Geometry: final body of the model. Coordinates: model frame, mm. Face numbers are marked on the shaded views. A direction names the side the tool comes from. Coordinates: 2 decimals unless noted, no trailing zeros. Write each loop counter-clockwise with the first axis right and the second up, starting at its lowest first coordinate (ties: lowest second). Pieces come first, ordered by that corner, then holes. Notation, with made-up numbers: (28, 46) -> (47, 46) arc R28 ccw to (47, 82) -> close; hole circle Ø3 at (32.5, 20). An arc over 180 degrees is marked (long way). One line per item, written item: value.
Autodesk Inventor part; units mm, degrees
ref_plane "YZ Plane" through (0, 0, 0) normal (1, 0, 0) x (0, 1, 0)
ref_plane "XZ Plane" through (0, 0, 0) normal (0, 1, 0) x (-1, 0, 0)
ref_plane "XY Plane" through (0, 0, 0) normal (0, 0, 1) x (1, 0, 0)
sketch "Sketch1" plane through (0, 0, 0) normal (1, 0, 0) x (0, 1, 0)
  arc A0 (-4.3875, 5.1282) -> (-5.1282, 4.3875) centre (0, 0) ccw
  arc A1 (-5.1895, 7.3532) -> (-4.3875, 5.1282) centre (-1.9912, 7.249) ccw
  arc A2 (-3.0589, 6.016) -> (-4.8075, 7.6084) centre (-5.9352, 4.6137) ccw
  arc A3 (-4.8075, 7.6084) -> (-5.1895, 7.3532) centre (0, 0) ccw
  arc A4 (-2.091, 6.4169) -> (-3.0589, 6.016) centre (0, 0) ccw
  arc A5 (-1.9805, 8.7794) -> (-2.091, 6.4169) centre (0.9345, 7.4592) ccw
  arc A6 (-1.5299, 8.869) -> (-1.9805, 8.7794) centre (0, 0) ccw
  arc A7 (-0.5238, 6.7286) -> (-1.5299, 8.869) centre (-3.7179, 6.5338) ccw
  arc A8 (0.5238, 6.7286) -> (-0.5238, 6.7286) centre (0, 0) ccw
  arc A9 (1.5299, 8.869) -> (0.5238, 6.7286) centre (3.7179, 6.5338) ccw
  arc A10 (1.9805, 8.7794) -> (1.5299, 8.869) centre (0, 0) ccw
  arc A11 (2.091, 6.4169) -> (1.9805, 8.7794) centre (-0.9345, 7.4592) ccw
  arc A12 (3.0589, 6.016) -> (2.091, 6.4169) centre (0, 0) ccw
  arc A13 (4.8075, 7.6084) -> (3.0589, 6.016) centre (5.9352, 4.6137) ccw
  arc A14 (5.1895, 7.3532) -> (4.8075, 7.6084) centre (0, 0) ccw
  arc A15 (4.3875, 5.1282) -> (5.1895, 7.3532) centre (1.9912, 7.249) ccw
  arc A16 (5.1282, 4.3875) -> (4.3875, 5.1282) centre (0, 0) ccw
  arc A17 (7.3532, 5.1895) -> (5.1282, 4.3875) centre (7.249, 1.9912) ccw
  arc A18 (7.6084, 4.8075) -> (7.3532, 5.1895) centre (0, 0) ccw
  arc A19 (6.016, 3.0589) -> (7.6084, 4.8075) centre (4.6137, 5.9352) ccw
  arc A20 (6.4169, 2.091) -> (6.016, 3.0589) centre (0, 0) ccw
  arc A21 (8.7794, 1.9805) -> (6.4169, 2.091) centre (7.4592, -0.9345) ccw
  arc A22 (8.869, 1.5299) -> (8.7794, 1.9805) centre (0, 0) ccw
  arc A23 (6.7286, 0.5238) -> (8.869, 1.5299) centre (6.5338, 3.7179) ccw
  arc A24 (6.7286, -0.5238) -> (6.7286, 0.5238) centre (0, 0) ccw
  arc A25 (8.869, -1.5299) -> (6.7286, -0.5238) centre (6.5338, -3.7179) ccw
  arc A26 (8.7794, -1.9805) -> (8.869, -1.5299) centre (0, 0) ccw
  arc A27 (6.4169, -2.091) -> (8.7794, -1.9805) centre (7.4592, 0.9345) ccw
  arc A28 (6.016, -3.0589) -> (6.4169, -2.091) centre (0, 0) ccw
  arc A29 (7.6084, -4.8075) -> (6.016, -3.0589) centre (4.6137, -5.9352) ccw
  arc A30 (7.3532, -5.1895) -> (7.6084, -4.8075) centre (0, 0) ccw
  arc A31 (5.1282, -4.3875) -> (7.3532, -5.1895) centre (7.249, -1.9912) ccw
  arc A32 (4.3875, -5.1282) -> (5.1282, -4.3875) centre (0, 0) ccw
  arc A33 (5.1895, -7.3532) -> (4.3875, -5.1282) centre (1.9912, -7.249) ccw
  arc A34 (4.8075, -7.6084) -> (5.1895, -7.3532) centre (0, 0) ccw
  arc A35 (3.0589, -6.016) -> (4.8075, -7.6084) centre (5.9352, -4.6137) ccw
  arc A36 (-8.869, 1.5299) -> (-6.7286, 0.5238) centre (-6.5338, 3.7179) ccw
  arc A37 (-6.7286, 0.5238) -> (-6.7286, -0.5238) centre (0, 0) ccw
  arc A38 (-6.7286, -0.5238) -> (-8.869, -1.5299) centre (-6.5338, -3.7179) ccw
  arc A39 (-8.869, -1.5299) -> (-8.7794, -1.9805) centre (0, 0) ccw
  arc A40 (-8.7794, -1.9805) -> (-6.4169, -2.091) centre (-7.4592, 0.9345) ccw
  arc A41 (-6.4169, -2.091) -> (-6.016, -3.0589) centre (0, 0) ccw
  arc A42 (-6.016, -3.0589) -> (-7.6084, -4.8075) centre (-4.6137, -5.9352) ccw
  arc A43 (-7.6084, -4.8075) -> (-7.3532, -5.1895) centre (0, 0) ccw
  arc A44 (-7.3532, -5.1895) -> (-5.1282, -4.3875) centre (-7.249, -1.9912) ccw
  arc A45 (-5.1282, -4.3875) -> (-4.3875, -5.1282) centre (0, 0) ccw
  arc A46 (-4.3875, -5.1282) -> (-5.1895, -7.3532) centre (-1.9912, -7.249) ccw
  arc A47 (-5.1895, -7.3532) -> (-4.8075, -7.6084) centre (0, 0) ccw
  arc A48 (-4.8075, -7.6084) -> (-3.0589, -6.016) centre (-5.9352, -4.6137) ccw
  arc A49 (-3.0589, -6.016) -> (-2.091, -6.4169) centre (0, 0) ccw
  arc A50 (-2.091, -6.4169) -> (-1.9805, -8.7794) centre (0.9345, -7.4592) ccw
  arc A51 (-1.9805, -8.7794) -> (-1.5299, -8.869) centre (0, 0) ccw
  arc A52 (-1.5299, -8.869) -> (-0.5238, -6.7286) centre (-3.7179, -6.5338) ccw
  arc A53 (-0.5238, -6.7286) -> (0.5238, -6.7286) centre (0, 0) ccw
  arc A54 (0.5238, -6.7286) -> (1.5299, -8.869) centre (3.7179, -6.5338) ccw
  arc A55 (1.5299, -8.869) -> (1.9805, -8.7794) centre (0, 0) ccw
  arc A56 (1.9805, -8.7794) -> (2.091, -6.4169) centre (-0.9345, -7.4592) ccw
  arc A57 (2.091, -6.4169) -> (3.0589, -6.016) centre (0, 0) ccw
  arc A58 (3.0589, -6.016) -> (4.8075, -7.6084) centre (5.9352, -4.6137) ccw
  arc A59 (4.8075, -7.6084) -> (5.1895, -7.3532) centre (0, 0) ccw
  arc A60 (5.1895, -7.3532) -> (4.3875, -5.1282) centre (1.9912, -7.249) ccw
  arc A61 (4.3875, -5.1282) -> (5.1282, -4.3875) centre (0, 0) ccw
  arc A62 (5.1282, -4.3875) -> (7.3532, -5.1895) centre (7.249, -1.9912) ccw
  arc A63 (7.3532, -5.1895) -> (7.6084, -4.8075) centre (0, 0) ccw
  arc A64 (7.6084, -4.8075) -> (6.016, -3.0589) centre (4.6137, -5.9352) ccw
  arc A65 (6.016, -3.0589) -> (6.4169, -2.091) centre (0, 0) ccw
  arc A66 (6.4169, -2.091) -> (8.7794, -1.9805) centre (7.4592, 0.9345) ccw
  arc A67 (8.7794, -1.9805) -> (8.869, -1.5299) centre (0, 0) ccw
  arc A68 (8.869, -1.5299) -> (6.7286, -0.5238) centre (6.5338, -3.7179) ccw
  arc A69 (6.7286, -0.5238) -> (6.7286, 0.5238) centre (0, 0) ccw
  arc A70 (6.7286, 0.5238) -> (8.869, 1.5299) centre (6.5338, 3.7179) ccw
  arc A71 (8.869, 1.5299) -> (8.7794, 1.9805) centre (0, 0) ccw
  arc A72 (8.7794, 1.9805) -> (6.4169, 2.091) centre (7.4592, -0.9345) ccw
  arc A73 (6.4169, 2.091) -> (6.016, 3.0589) centre (0, 0) ccw
  arc A74 (6.016, 3.0589) -> (7.6084, 4.8075) centre (4.6137, 5.9352) ccw
  arc A75 (7.6084, 4.8075) -> (7.3532, 5.1895) centre (0, 0) ccw
  arc A76 (7.3532, 5.1895) -> (5.1282, 4.3875) centre (7.249, 1.9912) ccw
  arc A77 (5.1282, 4.3875) -> (4.3875, 5.1282) centre (0, 0) ccw
  arc A78 (4.3875, 5.1282) -> (5.1895, 7.3532) centre (1.9912, 7.249) ccw
  arc A79 (5.1895, 7.3532) -> (4.8075, 7.6084) centre (0, 0) ccw
  arc A80 (4.8075, 7.6084) -> (3.0589, 6.016) centre (5.9352, 4.6137) ccw
  arc A81 (3.0589, 6.016) -> (2.091, 6.4169) centre (0, 0) ccw
  arc A82 (2.091, 6.4169) -> (1.9805, 8.7794) centre (-0.9345, 7.4592) ccw
  arc A83 (1.9805, 8.7794) -> (1.5299, 8.869) centre (0, 0) ccw
  arc A84 (1.5299, 8.869) -> (0.5238, 6.7286) centre (3.7179, 6.5338) ccw
  arc A85 (0.5238, 6.7286) -> (-0.5238, 6.7286) centre (0, 0) ccw
  arc A86 (-0.5238, 6.7286) -> (-1.5299, 8.869) centre (-3.7179, 6.5338) ccw
  arc A87 (-1.5299, 8.869) -> (-1.9805, 8.7794) centre (0, 0) ccw
  arc A88 (-1.9805, 8.7794) -> (-2.091, 6.4169) centre (0.9345, 7.4592) ccw
  arc A89 (-2.091, 6.4169) -> (-3.0589, 6.016) centre (0, 0) ccw
  arc A90 (-3.0589, 6.016) -> (-4.8075, 7.6084) centre (-5.9352, 4.6137) ccw
  arc A91 (-4.8075, 7.6084) -> (-5.1895, 7.3532) centre (0, 0) ccw
  arc A92 (-5.1895, 7.3532) -> (-4.3875, 5.1282) centre (-1.9912, 7.249) ccw
  arc A93 (-4.3875, 5.1282) -> (-5.1282, 4.3875) centre (0, 0) ccw
  arc A94 (-5.1282, 4.3875) -> (-7.3532, 5.1895) centre (-7.249, 1.9912) ccw
  arc A95 (-7.3532, 5.1895) -> (-7.6084, 4.8075) centre (0, 0) ccw
  arc A96 (-7.6084, 4.8075) -> (-6.016, 3.0589) centre (-4.6137, 5.9352) ccw
  arc A97 (-6.016, 3.0589) -> (-6.4169, 2.091) centre (0, 0) ccw
  arc A98 (-6.4169, 2.091) -> (-8.7794, 1.9805) centre (-7.4592, -0.9345) ccw
  arc A99 (-8.7794, 1.9805) -> (-8.869, 1.5299) centre (0, 0) ccw
  circle A100 centre (0, 0) radius 2.5
  line L0 (0, 0) -> (2.25, 0)
  line L1 (-1.5245, 0) -> (0, 0)
  line L2 (0, 0) -> (0, -2.5981)
  point P0 (3.0589, -6.016)
  point P1 (-5.1282, 4.3875)
  dimension "d17" = 5
extrude "Extrusion1" add sketch "Sketch1" along normal blind 4.5
sketch "Sketch4" plane through (4.5, 0, 0) normal (1, 0, 0) x (0, 0, -1)
  circle A0 centre (0, 0) radius 1.5
  arc A1 (6.016, 3.0589) -> (7.6084, 4.8075) centre (4.6137, 5.9352) ccw
  arc A2 (7.6084, 4.8075) -> (7.3532, 5.1895) centre (0, 0) ccw
  arc A3 (7.3532, 5.1895) -> (5.1282, 4.3875) centre (7.249, 1.9912) ccw
  arc A4 (5.1282, 4.3875) -> (4.3875, 5.1282) centre (0, 0) ccw
  arc A5 (4.3875, 5.1282) -> (5.1895, 7.3532) centre (1.9912, 7.249) ccw
  arc A6 (5.1895, 7.3532) -> (4.8075, 7.6084) centre (0, 0) ccw
  arc A7 (4.8075, 7.6084) -> (3.0589, 6.016) centre (5.9352, 4.6137) ccw
  arc A8 (3.0589, 6.016) -> (2.091, 6.4169) centre (0, 0) ccw
  arc A9 (2.091, 6.4169) -> (1.9805, 8.7794) centre (-0.9345, 7.4592) ccw
  arc A10 (1.9805, 8.7794) -> (1.5299, 8.869) centre (0, 0) ccw
  arc A11 (1.5299, 8.869) -> (0.5238, 6.7286) centre (3.7179, 6.5338) ccw
  arc A12 (0.5238, 6.7286) -> (-0.5238, 6.7286) centre (0, 0) ccw
  arc A13 (-0.5238, 6.7286) -> (-1.5299, 8.869) centre (-3.7179, 6.5338) ccw
  arc A14 (-1.5299, 8.869) -> (-1.9805, 8.7794) centre (0, 0) ccw
  arc A15 (-1.9805, 8.7794) -> (-2.091, 6.4169) centre (0.9345, 7.4592) ccw
  arc A16 (-2.091, 6.4169) -> (-3.0589, 6.016) centre (0, 0) ccw
  arc A17 (-3.0589, 6.016) -> (-4.8075, 7.6084) centre (-5.9352, 4.6137) ccw
  arc A18 (-4.8075, 7.6084) -> (-5.1895, 7.3532) centre (0, 0) ccw
  arc A19 (-5.1895, 7.3532) -> (-4.3875, 5.1282) centre (-1.9912, 7.249) ccw
  arc A20 (-4.3875, 5.1282) -> (-5.1282, 4.3875) centre (0, 0) ccw
  arc A21 (-5.1282, 4.3875) -> (-7.3532, 5.1895) centre (-7.249, 1.9912) ccw
  arc A22 (-7.3532, 5.1895) -> (-7.6084, 4.8075) centre (0, 0) ccw
  arc A23 (-7.6084, 4.8075) -> (-6.016, 3.0589) centre (-4.6137, 5.9352) ccw
  arc A24 (-6.016, 3.0589) -> (-6.4169, 2.091) centre (0, 0) ccw
  arc A25 (-6.4169, 2.091) -> (-8.7794, 1.9805) centre (-7.4592, -0.9345) ccw
  arc A26 (-8.7794, 1.9805) -> (-8.869, 1.5299) centre (0, 0) ccw
  arc A27 (-8.869, 1.5299) -> (-6.7286, 0.5238) centre (-6.5338, 3.7179) ccw
  arc A28 (-6.7286, 0.5238) -> (-6.7286, -0.5238) centre (0, 0) ccw
  arc A29 (-6.7286, -0.5238) -> (-8.869, -1.5299) centre (-6.5338, -3.7179) ccw
  arc A30 (-8.869, -1.5299) -> (-8.7794, -1.9805) centre (0, 0) ccw
  arc A31 (-8.7794, -1.9805) -> (-6.4169, -2.091) centre (-7.4592, 0.9345) ccw
  arc A32 (-6.4169, -2.091) -> (-6.016, -3.0589) centre (0, 0) ccw
  arc A33 (-6.016, -3.0589) -> (-7.6084, -4.8075) centre (-4.6137, -5.9352) ccw
  arc A34 (-7.6084, -4.8075) -> (-7.3532, -5.1895) centre (0, 0) ccw
  arc A35 (-7.3532, -5.1895) -> (-5.1282, -4.3875) centre (-7.249, -1.9912) ccw
  arc A36 (-5.1282, -4.3875) -> (-4.3875, -5.1282) centre (0, 0) ccw
  arc A37 (-4.3875, -5.1282) -> (-5.1895, -7.3532) centre (-1.9912, -7.249) ccw
  arc A38 (-5.1895, -7.3532) -> (-4.8075, -7.6084) centre (0, 0) ccw
  arc A39 (-4.8075, -7.6084) -> (-3.0589, -6.016) centre (-5.9352, -4.6137) ccw
  arc A40 (-3.0589, -6.016) -> (-2.091, -6.4169) centre (0, 0) ccw
  arc A41 (-2.091, -6.4169) -> (-1.9805, -8.7794) centre (0.9345, -7.4592) ccw
  arc A42 (-1.9805, -8.7794) -> (-1.5299, -8.869) centre (0, 0) ccw
  arc A43 (-1.5299, -8.869) -> (-0.5238, -6.7286) centre (-3.7179, -6.5338) ccw
  arc A44 (-0.5238, -6.7286) -> (0.5238, -6.7286) centre (0, 0) ccw
  arc A45 (0.5238, -6.7286) -> (1.5299, -8.869) centre (3.7179, -6.5338) ccw
  arc A46 (1.5299, -8.869) -> (1.9805, -8.7794) centre (0, 0) ccw
  arc A47 (1.9805, -8.7794) -> (2.091, -6.4169) centre (-0.9345, -7.4592) ccw
  arc A48 (2.091, -6.4169) -> (3.0589, -6.016) centre (0, 0) ccw
  arc A49 (3.0589, -6.016) -> (4.8075, -7.6084) centre (5.9352, -4.6137) ccw
  arc A50 (4.8075, -7.6084) -> (5.1895, -7.3532) centre (0, 0) ccw
  arc A51 (5.1895, -7.3532) -> (4.3875, -5.1282) centre (1.9912, -7.249) ccw
  arc A52 (4.3875, -5.1282) -> (5.1282, -4.3875) centre (0, 0) ccw
  arc A53 (5.1282, -4.3875) -> (7.3532, -5.1895) centre (7.249, -1.9912) ccw
  arc A54 (7.3532, -5.1895) -> (7.6084, -4.8075) centre (0, 0) ccw
  arc A55 (7.6084, -4.8075) -> (6.016, -3.0589) centre (4.6137, -5.9352) ccw
  arc A56 (6.016, -3.0589) -> (6.4169, -2.091) centre (0, 0) ccw
  arc A57 (6.4169, -2.091) -> (8.7794, -1.9805) centre (7.4592, 0.9345) ccw
  arc A58 (8.7794, -1.9805) -> (8.869, -1.5299) centre (0, 0) ccw
  arc A59 (8.869, -1.5299) -> (6.7286, -0.5238) centre (6.5338, -3.7179) ccw
  arc A60 (6.7286, -0.5238) -> (6.7286, 0.5238) centre (0, 0) ccw
  arc A61 (6.7286, 0.5238) -> (8.869, 1.5299) centre (6.5338, 3.7179) ccw
  arc A62 (8.869, 1.5299) -> (8.7794, 1.9805) centre (0, 0) ccw
  arc A63 (8.7794, 1.9805) -> (6.4169, 2.091) centre (7.4592, -0.9345) ccw
  arc A64 (6.4169, 2.091) -> (6.016, 3.0589) centre (0, 0) ccw
  circle A65 centre (0, 0) radius 2.5
  circle A66 centre (0, 0) radius 3
  dimension "d18" = 3
  dimension "d19" = 6
extrude "Extrusion3" add sketch "Sketch4" along normal blind 2 contours A65 | A66
fillet "Fillet1" radius 1 1 edges at (4.5, 0, 3)
equation "\"d17\" = d_agu"
equation "\"d_agu\" = 5"
properties part number "engrane_v3"
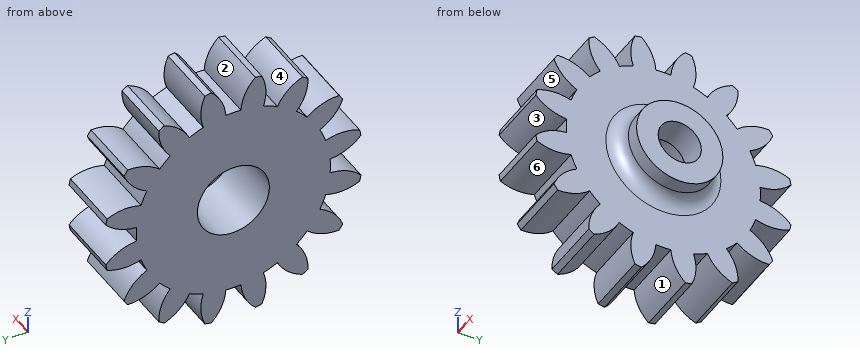
(1) Reachability of the marked faces 4, 5 and 6 from +Z, -Z, +X, -X, +Y, -Y: full face, straight path, thin tool, end or side. Return the list, or none.
Responses:
face 4: +Z, +X, -X
face 5: +X, -X, -Y
face 6: +X, -X
(2) First-contact query: pin 1 (1.5 mm diameter, centred on x = 2, z = 6.5, fed in from -Y); pin 2 (1.5 mm diameter, centred on x = 2, z = -4, fed in from +Y). Flat tips, straight axial feed; report the tip coordinate or a pass-through.
Responses:
pin 1: stops at y = -5.19
pin 2: stops at y = 7.59
(3) Pull-direction query (Z, two-part tool) for the marked faces 1, 2 and 3; classes: released by +Z, released by -Z, zero draft, split by the parting line, or undercut.
Responses:
face 1: released by -Z
face 2: released by +Z
face 3: undercut
(4) Line query: line 1 (Y direction, x = 5.8, z = 0); line 2 (Y direction, x = 1, z = 4.75); line 3 (Y direction, x = 0.5, z = 7). Output: solid intervals per line, ascending. Write a range as [from, to].
Responses:
line 1: y = [-3, -1.5], [1.5, 3]
line 2: y = [-7.59, -5.63], [-4.79, 4.79], [5.63, 7.59]
line 3: y = [-5.18, -3.8], [-2.23, -0.55], [0.55, 2.23], [3.8, 5.18]
(5) Section A-A (y = 0). Return the cut outline in (x, z).
Responses:
outline: (0, -6.75) -> (4.5, -6.75) -> (4.5, -4) arc R1 cw to (5.5, -3) -> (6.5, -3) -> (6.5, -1.5) -> (4.5, -1.5) -> (4.5, -2.5) -> (0, -2.5) -> close; (0, 2.5) -> (4.5, 2.5) -> (4.5, 1.5) -> (6.5, 1.5) -> (6.5, 3) -> (5.5, 3) arc R1 cw to (4.5, 4) -> (4.5, 6.75) -> (0, 6.75) -> close
(6) Section C-C (x = 5). Return the cut outline in (y, z).
Responses:
outline: circle Ø6.27 at (0, 0); hole circle Ø3 at (0, 0)
